For this review, take the finished solid that the model builds, in its own axes (mm). A direction names the side the tool comes from. Give positions to 0.01 mm unless a question says otherwise; leave off trailing zeros. Loops run counter-clockwise (first coordinate to the right, second up) from the corner with the lowest first, then second, coordinate; pieces in that order, holes last. Notation, with made-up numbers: (10, 70.5) - (14, 70.5) arc R17 cw to (14, 77.5) - close; hole circle Ø7 at (-24.75, 11). An arc over 180 degrees is marked (long way). Put each result on its own line as item: value. Start each with the question number.
from build123d import *

# Parameters (mm, degrees)
BOSS_EXTRUDE1_DEPTH = 12.7
FILLET1_R           = 6.35
SKETCH2_R           = 3.81
CUT_EXTRUDE1_DEPTH  = 327.762880389
SKETCH3_R           = 3.81
CUT_EXTRUDE2_DEPTH  = 327.762880389


with BuildPart() as part:
    # Sketch1 → Boss-Extrude1 (new body)
    with BuildSketch(Plane(origin=(0, 0, 0), x_dir=(1, 0, 0), z_dir=(0, 1, 0))):
        with BuildLine():
            Line((0, 0), (12.7, 0))
            Line((12.7, 0), (12.7, -25.4))
            ThreePointArc((12.7, -25.4), (20.139487758, -43.360512242), (38.1, -50.8))
            ThreePointArc((38.1, -50.8), (56.060512242, -43.360512242), (63.5, -25.4))
            Line((63.5, -25.4), (63.5, 0))
            Line((63.5, 0), (76.2, 0))
            Line((76.2, 0), (76.2, -50.8))
            ThreePointArc((76.2, -50.8), (55.181226716, -158.75), (76.2, -266.7))
            Line((76.2, -266.7), (76.2, -317.5))
            Line((76.2, -317.5), (63.5, -317.5))
            Line((63.5, -317.5), (63.5, -292.1))
            ThreePointArc((63.5, -292.1), (56.060512242, -274.139487758), (38.1, -266.7))
            ThreePointArc((38.1, -266.7), (20.139487758, -274.139487758), (12.7, -292.1))
            Line((12.7, -292.1), (12.7, -317.5))
            Line((12.7, -317.5), (0, -317.5))
            Line((0, -317.5), (0, -266.7))
            ThreePointArc((0, -266.7), (21.018773284, -158.75), (0, -50.8))
            Line((0, -50.8), (0, 0))
        make_face()
    extrude(amount=BOSS_EXTRUDE1_DEPTH)

    # Fillet1
    fillet1_edges = [part.edges().sort_by_distance(p)[0] for p in [
        (69.85, 0, 0),
        (6.35, 0, 0),
        (69.85, 12.7, 0),
        (6.35, 12.7, 0),
        (6.35, 0, 317.5),
        (6.35, 12.7, 317.5),
        (69.85, 0, 317.5),
        (69.85, 12.7, 317.5),
    ]]
    fillet(fillet1_edges, radius=FILLET1_R - 0.0001)  # a hair under: the kernel refuses the full size

    # Sketch2 → Cut-Extrude1 (cut, through all)
    with BuildSketch(Plane(origin=(76.2, 0, 0), x_dir=(0, 0, -1), z_dir=(1, 0, 0))):
        with Locations((-311.15, 6.35)):
            Circle(SKETCH2_R)
    extrude(amount=-CUT_EXTRUDE1_DEPTH, mode=Mode.SUBTRACT)

    # Sketch3 → Cut-Extrude2 (cut, through all)
    with BuildSketch(Plane(origin=(76.2, 0, 0), x_dir=(0, 0, -1), z_dir=(1, 0, 0))):
        with Locations((-6.35, 6.35)):
            Circle(SKETCH3_R)
    extrude(amount=-CUT_EXTRUDE2_DEPTH, mode=Mode.SUBTRACT)


solid = part.part
1) Wall thickness on probe 1 along Y at (x, z) = (70.25, 6.35); probe 2 along X at (y, z) = (11.25, 291); probe 3 along X at (y, z) = (6.25, 163.5): over which ranges is each line inside the solid? List them lowest first.
2) Take a section at D-D on z = 253. State the section outline as (x, y) points.
3) Take a section at B-B on x = 59. State the section outline as (y, z) points.
4) Machinability: for faces 5 (the flat face through (39, 0, 157)), 6 (the flat face through (12.7, 6, 15)), which of the approach directions +Z, -Z, +X, -X, +Y, -Y give a long, thin tool a straight path to every point of the face, cutting with its end or side? Answer none if there is none.
5) Take a section at C-C on z = 171. State the section outline as (x, y) points, and give its area (3 significant figures).
6) Mouldability with a two-part tool opening along X and no side actions: class faces 1 (the flat face through (12.7, 6, 302)), 2 (the cylindrical face through (6.439, 6.518, 314.956)), 3 (the cylindrical face through (55.185, 6.261, 157.201)), 4 (the flat face through (63.5, 6, 302)) as released by +X, released by -X, zero draft, split by the parting line, or undercut.
7) Take a section at A-A on z = 31. State the section outline as (x, y) points, and give its area (3 significant figures).
8) Insertion check: P1, Ø2, axis at x = 36, y = 4, coming from the +Z side; P2, Ø4, axis at y = 2, z = 230.5, coming from the -X side; P3, Ø6, axis at x = 48.5, y = 3.5, coming from the +Z side. Each pin has a flat end and moves straight along its axis. Give the tip position at first contact, or say it passes through.
Answers follow:
1. probe 1: 0 to 2.54, 10.16 to 12.7
1. probe 2: 0 to 12.72, 63.48 to 76.2
1. probe 3: 20.98 to 55.22
2. outline: (5.14, 0) - (71.06, 0) - (71.06, 12.7) - (5.14, 12.7) - close
3. outline: (0, 39.83) - (12.7, 39.83) - (12.7, 112.03) - (0, 112.03) - close; (0, 205.47) - (12.7, 205.47) - (12.7, 277.67) - (0, 277.67) - close
4. face 5: +Z, -Z, +X, -X, -Y
4. face 6: -Z, +Y, -Y
5. outline: (20.76, 0) - (55.44, 0) - (55.44, 12.7) - (20.76, 12.7) - close
5. area: 440 mm2
6. face 1: undercut
6. face 2: zero draft
6. face 3: released by +X
6. face 4: undercut
7. outline: (0, 0) - (13.33, 0) - (13.33, 12.7) - (0, 12.7) - close; (62.87, 0) - (76.2, 0) - (76.2, 12.7) - (62.87, 12.7) - close
7. area: 338 mm2
8. P1: z = 266.89
8. P2: x = 11.41
8. P3: z = 270.52
